from build123d import *

# Parameters (mm, degrees)
EXTRUDE_1_DEPTH     = 3
SKETCH_4_W          = 70
SKETCH_4_H          = 3
EXTRUDE_2_DEPTH     = 9.25
CUT_EXTRUDE_1_REACH = 91.308
SKETCH_5_R          = 1.65
FILLET_1_R          = 1
EXTRUDE_3_DEPTH     = 5
CUT_EXTRUDE_2_REACH = 91.308


with BuildPart() as part:
    # ｽｹｯﾁ2 → ﾎﾞｽ - 押し出し1 (new body)
    with BuildSketch(Plane(origin=(0, 0, 0), x_dir=(1, 0, 0), z_dir=(0, 1, 0))):
        with BuildLine():
            Line((70, 7.6), (40, 7.6))
            Line((40, 7.6), (40, 4.4))
            Line((40, 4.4), (70, 4.4))
            Line((70, 4.4), (87.5, 4.4))
            ThreePointArc((87.5, 4.4), (87.853553391, 4.253553391), (88, 3.9))
            Line((88, 3.9), (88, 0.5))
            ThreePointArc((88, 0.5), (87.853553391, 0.146446609), (87.5, 0))
            Line((87.5, 0), (85.383249581, 0))
            ThreePointArc((85.383249581, 0), (78.75, 2), (72.116750419, 0))
            Line((72.116750419, 0), (70, 0))
            Line((70, 0), (62, 0))
            Line((62, 0), (62, -0.949194177))
            ThreePointArc((62, -0.949194177), (61.80461807, -1.345688605), (61.371168675, -1.432311647))
            Line((61.371168675, -1.432311647), (56, 0))
            Line((56, 0), (0.5, 0))
            ThreePointArc((0.5, 0), (0.146446609, 0.146446609), (0, 0.5))
            Line((0, 0.5), (0, 11.5))
            ThreePointArc((0, 11.5), (0.146446609, 11.853553391), (0.5, 12))
            Line((0.5, 12), (70, 12))
            Line((70, 12), (72.116750419, 12))
            ThreePointArc((72.116750419, 12), (78.75, 10), (85.383249581, 12))
            Line((85.383249581, 12), (87.5, 12))
            ThreePointArc((87.5, 12), (87.853553391, 11.853553391), (88, 11.5))
            Line((88, 11.5), (88, 8.1))
            ThreePointArc((88, 8.1), (87.853553391, 7.746446609), (87.5, 7.6))
            Line((87.5, 7.6), (70, 7.6))
        make_face()
    extrude(amount=EXTRUDE_1_DEPTH)

    # ｽｹｯﾁ4 → ﾎﾞｽ - 押し出し2 (add)
    with BuildSketch(Plane(origin=(0, 3, 0), x_dir=(1, 0, 0), z_dir=(0, 1, 0))):
        with Locations((35, 9.1)):
            Rectangle(SKETCH_4_W, SKETCH_4_H)
    extrude(amount=EXTRUDE_2_DEPTH)

    # ｽｹｯﾁ5 → ｶｯﾄ - 押し出し1 (cut, up to next)
    with BuildSketch(Plane.XY.offset(-7.6), mode=Mode.PRIVATE) as cut_extrude_1_sk1:
        with Locations((3.45, 8.95)):
            Circle(SKETCH_5_R)
    cut_extrude_1_tool1 = extrude(cut_extrude_1_sk1.sketch, amount=-CUT_EXTRUDE_1_REACH, mode=Mode.PRIVATE) & part.part
    # ｽｹｯﾁ5 → ｶｯﾄ - 押し出し1 (cut, up to next)
    with BuildSketch(Plane.XY.offset(-7.6), mode=Mode.PRIVATE) as cut_extrude_1_sk2:
        with Locations((66.55, 8.95)):
            Circle(SKETCH_5_R)
    cut_extrude_1_tool2 = extrude(cut_extrude_1_sk2.sketch, amount=-CUT_EXTRUDE_1_REACH, mode=Mode.PRIVATE) & part.part
    add(cut_extrude_1_tool1.solids().sort_by_distance((3.45, 8.95, -7.6))[0], mode=Mode.SUBTRACT)
    add(cut_extrude_1_tool2.solids().sort_by_distance((66.55, 8.95, -7.6))[0], mode=Mode.SUBTRACT)

    # ﾌｨﾚｯﾄ1
    fillet_1_edges = [part.edges().sort_by_distance(p)[0] for p in [
        (70, 12.25, -9.1),
        (0, 12.25, -9.1),
    ]]
    fillet(fillet_1_edges, radius=FILLET_1_R)

    # ｽｹｯﾁ6 → ﾎﾞｽ - 押し出し3 (add)
    with BuildSketch(Plane(origin=(0, 3, 0), x_dir=(1, 0, 0), z_dir=(0, 1, 0))):
        with BuildLine():
            Line((88, 11.5), (88, 8.1))
            ThreePointArc((88, 8.1), (87.853553391, 7.746446609), (87.5, 7.6))
            Line((87.5, 7.6), (72.116750419, 7.6))
            ThreePointArc((72.116750419, 7.6), (71.763197029, 7.746446609), (71.616750419, 8.1))
            Line((71.616750419, 8.1), (71.616750419, 11.5))
            ThreePointArc((71.616750419, 11.5), (71.763197029, 11.853553391), (72.116750419, 12))
            ThreePointArc((72.116750419, 12), (78.75, 10), (85.383249581, 12))
            Line((85.383249581, 12), (87.5, 12))
            ThreePointArc((87.5, 12), (87.853553391, 11.853553391), (88, 11.5))
        make_face()
        with BuildLine():
            Line((88, 3.9), (88, 0.5))
            ThreePointArc((88, 0.5), (87.853553391, 0.146446609), (87.5, 0))
            Line((87.5, 0), (85.383249581, 0))
            ThreePointArc((85.383249581, 0), (78.75, 2), (72.116750419, 0))
            ThreePointArc((72.116750419, 0), (71.763197029, 0.146446609), (71.616750419, 0.5))
            Line((71.616750419, 0.5), (71.616750419, 3.9))
            ThreePointArc((71.616750419, 3.9), (71.763197029, 4.253553391), (72.116750419, 4.4))
            Line((72.116750419, 4.4), (87.5, 4.4))
            ThreePointArc((87.5, 4.4), (87.853553391, 4.253553391), (88, 3.9))
        make_face()
    extrude(amount=EXTRUDE_3_DEPTH)

    # ｽｹｯﾁ7 → ｶｯﾄ - 押し出し2 (cut, up to next)
    with BuildSketch(Plane.XY.offset(-7.6), mode=Mode.PRIVATE) as cut_extrude_2_sk1:
        Polygon((8, 12.25), (12, 10.25), (58, 10.25), (62, 12.25), align=None)
    cut_extrude_2_tool1 = extrude(cut_extrude_2_sk1.sketch, amount=-CUT_EXTRUDE_2_REACH, mode=Mode.PRIVATE) & part.part
    add(cut_extrude_2_tool1.solids().sort_by_distance((35, 11.276667, -7.6))[0], mode=Mode.SUBTRACT)


solid = part.part
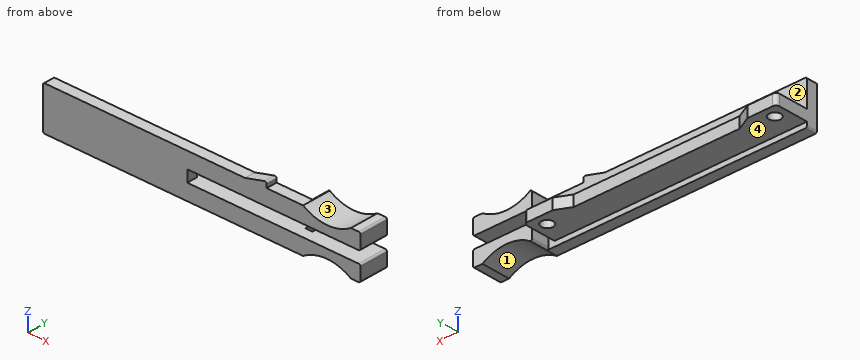
The listing builds one solid part. Answer for the finished solid, in the listing's coordinates (mm). Face numbers are marked on the shaded views. A direction names the side the tool comes from. Give positions to 0.01 mm unless a question says otherwise; leave off trailing zeros. Write each loop counter-clockwise with the first axis right and the second up, starting at its lowest first coordinate (ties: lowest second). Pieces come first, ordered by that corner, then holes.
1) Section D-D (z = -6) is taken. Write down the section's boundary in (x, y), and give its area (3 significant figures).
2) For a pull along X with two mould halves and no side action, classify the marked faces 3 and 4 as pulls with the +X half, pulls with the -X half, needs draft (parallel to the pull), parting line crosses it, or undercut.
3) Given P1, Ø1, axis at x = 71, z = -5, coming from the +Y side; P2, Ø6, axis at x = 62.5, y = 5, coming from the +Z side; P3, Ø1, axis at y = 4.5, z = -1.5, coming from the -X side; P4, Ø5, axis at x = 53, z = -10, coming from the +Y side, each flat-ended and moving along its own axis, determine where each tip first touches the part or whether it passes through.
4) A tool of negligible diameter and unlimited length cuts with its end or side. For the marked faces 1 and 2, from which of +Z, -Z, +X, -X, +Y, -Y can it reach the whole face along a straight path? Write none if from no direction.
5) Find the intervals of material crossed by L1, parallel to Y at x = 66.55, z = -8.3; L2, parallel to Z at x = 34, y = 6.5; L3, parallel to Y at x = 84, z = -9.75, in increasing order.
6) Section C-C (x = 66.55) is taken. Write down the section's boundary in (y, z), and give its area (4 significant figures).
7) Section A-A (y = 6) is taken. Write down the section's boundary in (x, z), and give its area (3 significant figures).
8) Section B-B (x = 3.45) is taken. Write down the section's boundary in (y, z), and give its area (4 significant figures).
Response:
1. outline: (0, 0) - (40, 0) - (40, 3) - (0, 3) - close
1. area: 120 mm2
2. face 3: undercut
2. face 4: needs draft
3. P1: passes through
3. P2: stops at z = 1.45
3. P3: stops at x = 71.62
3. P4: stops at y = 10.25
4. face 1: -Z, +Y, -Y
4. face 2: +Z, -X, +Y
5. L1: y = 0 to 7.3, 10.6 to 12.25
5. L2: z = -10.6 to -7.6
5. L3: y = 0 to 8
6. outline: (0, -12) - (3, -12) - (3, -10.6) - (7.3, -10.6) - (7.3, -7.6) - (0, -7.6) - close; (0, -4.4) - (3, -4.4) - (3, 0) - (0, 0) - close; (10.6, -10.6) - (12.25, -10.6) - (12.25, -7.6) - (10.6, -7.6) - close
6. area: 44.25 mm2
7. outline: (0, -10.6) - (70, -10.6) - (70, -7.6) - (0, -7.6) - close; (71.62, -11.5) arc R0.5 ccw to (72.12, -12) arc R12 cw to (85.38, -12) - (87.5, -12) arc R0.5 ccw to (88, -11.5) - (88, -8.1) arc R0.5 ccw to (87.5, -7.6) - (72.12, -7.6) arc R0.5 ccw to (71.62, -8.1) - close; (71.62, -3.9) arc R0.5 ccw to (72.12, -4.4) - (87.5, -4.4) arc R0.5 ccw to (88, -3.9) - (88, -0.5) arc R0.5 ccw to (87.5, 0) - (85.38, 0) arc R12 cw to (72.12, 0) arc R0.5 ccw to (71.62, -0.5) - close
7. area: 318 mm2
8. outline: (0, -12) - (3, -12) - (3, -10.6) - (7.3, -10.6) - (7.3, -7.6) - (3, -7.6) - (3, 0) - (0, 0) - close; (10.6, -10.6) - (12.25, -10.6) - (12.25, -7.6) - (10.6, -7.6) - close
8. area: 53.85 mm2
